Could you check a few things on this model? Use its own coordinates, in mm. A direction names the side the tool comes from. Round coordinates to 2 decimals unless told otherwise and drop trailing zeros. Loops run counter-clockwise (first coordinate to the right, second up) from the corner with the lowest first, then second, coordinate; pieces in that order, holes last. Notation, with made-up numbers: (47.25, 70.25) -> (68.25, 70.25) arc R25 ccw to (68.25, 101.25) -> close; hole circle Ø10 at (67, 1.25). An arc over 180 degrees is marked (long way). One line per item, written item: value.
```python
from build123d import *

# Parameters (mm, degrees)
SKETCH1_W                      = 22
SKETCH1_H                      = 2.4
SKETCH2_R                      = 11
BOSS_EXTRUDE1_DEPTH            = 5
SKETCH3_R                      = 3.9
BOSS_EXTRUDE2_DEPTH            = 9
SKETCH4_R                      = 11
BOSS_EXTRUDE3_DEPTH            = 20.6
SKETCH5_W                      = 0.25
SKETCH5_H                      = 10
SKETCH6_W                      = 0.25
SKETCH6_H                      = 10
SKETCH7_W                      = 0.25
SKETCH7_H                      = 10
SKETCH8_W                      = 0.25
SKETCH8_H                      = 10
SKETCH9_W                      = 0.25
SKETCH9_H                      = 10
SKETCH10_W                     = 0.25
SKETCH10_H                     = 10
SKETCH11_W                     = 0.25
SKETCH11_H                     = 10
SKETCH12_W                     = 0.25
SKETCH12_H                     = 10
F_5_5_5_5_DIAMETER_HOLE1_D     = 5.5
F_5_5_5_5_DIAMETER_HOLE1_DEPTH = 26.4


with BuildPart() as part:
    # Sketch1 → Revolve1 (revolve)
    with BuildSketch(Plane.XZ):
        with Locations((11, 1.2)):
            Rectangle(SKETCH1_W, SKETCH1_H)
    revolve(axis=Axis((0, 0, 2.4), (0, 0, -1)))

    # Sketch2 → Boss-Extrude1 (add)
    with BuildSketch(Plane.XY.offset(2.4)):
        Circle(SKETCH2_R)
    extrude(amount=BOSS_EXTRUDE1_DEPTH)

    # Sketch3 → Boss-Extrude2 (add)
    with BuildSketch(Plane.XY.offset(7.4)):
        Circle(SKETCH3_R)
    extrude(amount=BOSS_EXTRUDE2_DEPTH)

    # Sketch4 → Boss-Extrude3 (add)
    with BuildSketch(Plane(origin=(0, 0, 0), x_dir=(-1, 0, 0), z_dir=(0, 0, -1))):
        Circle(SKETCH4_R)
    extrude(amount=BOSS_EXTRUDE3_DEPTH)

    # Sketch5 → Revolve2 (revolve)
    with BuildSketch(Plane.XZ.offset(0.675788748)):
        with Locations((0.22311943, 21.4)):
            Rectangle(SKETCH5_W, SKETCH5_H)
    revolve(axis=Axis((0.09811943, -0.675788748, 26.4), (0, 0, -1)))

    # Sketch6 → Revolve3 (revolve)
    with BuildSketch(Plane.XZ.offset(-0.091161083)):
        with Locations((-0.260169312, 21.4)):
            Rectangle(SKETCH6_W, SKETCH6_H)
    revolve(axis=Axis((-0.385169312, 0.091161083, 26.4), (0, 0, -1)))

    # Sketch7 → Revolve4 (revolve)
    with BuildSketch(Plane.XZ.offset(0.562471217)):
        with Locations((-0.402355812, 21.4)):
            Rectangle(SKETCH7_W, SKETCH7_H)
    revolve(axis=Axis((-0.527355812, -0.562471217, 26.4), (0, 0, -1)))

    # Sketch8 → Revolve5 (revolve)
    with BuildSketch(Plane(origin=(0, 0, 0), x_dir=(1, 0, 0), z_dir=(0, 1, 0))):
        with Locations((-9.138912968, 25.6)):
            Rectangle(SKETCH8_W, SKETCH8_H)
    revolve(axis=Axis((-9.263912968, 0, -30.6), (0, 0, 1)))

    # Sketch9 → Revolve6 (revolve)
    with BuildSketch(Plane(origin=(0, 0, 0), x_dir=(1, 0, 0), z_dir=(0, 1, 0))):
        with Locations((10.149169803, 25.6)):
            Rectangle(SKETCH9_W, SKETCH9_H)
    revolve(axis=Axis((10.024169803, 0, -30.6), (0, 0, 1)))

    # Sketch10 → Revolve7 (revolve)
    with BuildSketch(Plane(origin=(0, 0, 0), x_dir=(1, 0, 0), z_dir=(0, 1, 0))):
        with Locations((9.469293537, 25.6)):
            Rectangle(SKETCH10_W, SKETCH10_H)
    revolve(axis=Axis((9.344293537, 0, -30.6), (0, 0, 1)))

    # Sketch11 → Revolve8 (revolve)
    with BuildSketch(Plane(origin=(0, 0, 0), x_dir=(1, 0, 0), z_dir=(0, 1, 0))):
        with Locations((-9.977336314, 25.6)):
            Rectangle(SKETCH11_W, SKETCH11_H)
    revolve(axis=Axis((-10.102336314, 0, -30.6), (0, 0, 1)))

    # Sketch12 → Revolve9 (revolve)
    with BuildSketch(Plane.XZ):
        with Locations((0.388776295, 21.4)):
            Rectangle(SKETCH12_W, SKETCH12_H)
    revolve(axis=Axis((0.263776295, 0, 26.4), (0, 0, -1)))

    # Ø5.5 (5.5) Diameter Hole1
    with Locations(Plane(origin=(0, 0, 0), x_dir=(-1, 0, 0), z_dir=(0, 0, -1))):
        with Locations((-15.155444566, 8.75), (15.155444566, 8.75), (0, -17.5)):
            Hole(F_5_5_5_5_DIAMETER_HOLE1_D / 2, depth=F_5_5_5_5_DIAMETER_HOLE1_DEPTH)


solid = part.part
```
Item 1: If we mould it in two halves opening along Y, with no side actions, what happens to faces 4 (the face through (-2.87, 2.64, 11.84)), 5 (the face through (-12.532, 9.576, 1.217)), 6 (the face through (0, -5, 7.4))? For each: released by +Y, released by -Y, zero draft, split by the parting line, or undercut.
Output:
face 4: split by the parting line
face 5: undercut
face 6: zero draft
Item 2: If we section it at C-C on x = 7.5: List the corners of the cut face in (y, z) for me, plus the area to 3 significant figures.
Output:
outline: (-20.68, 0) -> (-8.05, 0) -> (-8.05, -20.6) -> (8.05, -20.6) -> (8.05, 0) -> (20.68, 0) -> (20.68, 2.4) -> (8.05, 2.4) -> (8.05, 7.4) -> (-8.05, 7.4) -> (-8.05, 2.4) -> (-20.68, 2.4) -> close
area: 511 mm²
Item 3: If we section it at A-A on y = -17.5: List the corners of the cut face in (x, z) for me.
Output:
outline: (-13.33, 0) -> (-2.75, 0) -> (-2.75, 2.4) -> (-13.33, 2.4) -> close; (2.75, 0) -> (13.33, 0) -> (13.33, 2.4) -> (2.75, 2.4) -> close
Item 4: For faces 1 (the face through (-2.38, -10.74, 4.86)), 2 (the face through (-0.358, -14.773, 1.217)), 3 (the face through (2.38, -10.74, -10.16)), which set-ups out of +Z, -Z, +X, -X, +Y, -Y let a thin tool reach every point of the face, with its end or its side?
Output:
face 1: +Z
face 2: +Z, -Z
face 3: -Z
Item 5: Will these pins go through, and if not, where does the flat tip stop? pin 1 Ø4.5 at (x, y) = (15.16, 8.75) entering from -Z; pin 2 Ø10 at (y, z) = (-7, -19) entering from -X; pin 3 Ø2 at (x, y) = (-13.5, 17) entering from +Z; pin 4 Ø3 at (y, z) = (-9.5, -6) entering from +X.
Output:
pin 1: passes through
pin 2: stops at x = -10.82
pin 3: stops at z = 2.4
pin 4: stops at x = 7.55
Item 6: I need wall thicknesses on line 1 (Y direction, x = 0, z = 0.7); line 2 (X direction, y = 8, z = 1); line 3 (Z direction, x = 20, y = -1). Which ranges of each line are inside material? Lowest first, please. Write a range as from..to.
Output:
line 1: y = -22..-20.25, -14.75..22
line 2: x = -20.49..-17.8, -12.51..12.51, 17.8..20.49
line 3: z = 0..2.4
Item 7: If we section it at B-B on y = 8.75: List the corners of the cut face in (x, z) for me.
Output:
outline: (-20.19, 0) -> (-17.91, 0) -> (-17.91, 2.4) -> (-20.19, 2.4) -> close; (-12.41, 0) -> (-6.67, 0) -> (-6.67, -20.6) -> (6.67, -20.6) -> (6.67, 0) -> (12.41, 0) -> (12.41, 2.4) -> (6.67, 2.4) -> (6.67, 7.4) -> (-6.67, 7.4) -> (-6.67, 2.4) -> (-12.41, 2.4) -> close; (17.91, 0) -> (20.19, 0) -> (20.19, 2.4) -> (17.91, 2.4) -> close
Item 8: If we section it at D-D on z = -11: List the corners of the cut face in (x, y) for me.
Output:
outline: circle Ø22 at (0, 0)
